CAD build for the part. Positions are in the model's coordinates, mm. Face numbers are marked on the shaded views. A direction names the side the tool comes from. Give positions to 0.01 mm unless a question says otherwise; leave off trailing zeros. Order: outer loops, then holes, each group sorted by start corner. A loop starts at its lowest first (then second) coordinate and runs counter-clockwise, first axis right, second up.
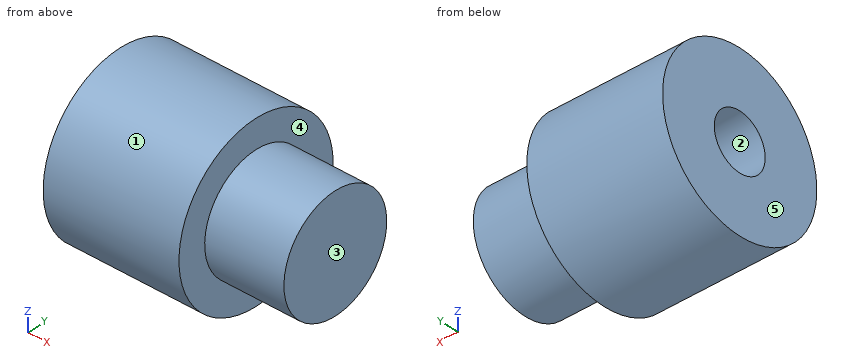
from build123d import *

# Parameters (mm, degrees)
SOCKET_1_SKETCH_W = 11.5
SOCKET_1_SKETCH_H = 4.953


with BuildPart() as part:
    # Reg_Outlet_Upper Sketch → Reg_Outlet_Upper (revolve)
    with BuildSketch(Plane.XY, mode=Mode.PRIVATE) as reg_outlet_upper_sk:
        Polygon((14, 0), (14, 10), (0, 10), (0, 15), (-24, 15), (-24, 0), align=None)
    revolve(reg_outlet_upper_sk.sketch.rotate(Axis((-1000, 0, 0), (1, 0, 0)), 90), axis=Axis((-1000, 0, 0), (1, 0, 0)))

    # Socket 1 Sketch → Socket 1 (revolve, cut)
    with BuildSketch(Plane.XY, mode=Mode.PRIVATE) as socket_1_sk:
        with Locations((-19.25, 2.4765)):
            Rectangle(SOCKET_1_SKETCH_W, SOCKET_1_SKETCH_H)
    revolve(socket_1_sk.sketch.rotate(Axis((-1000, 0, 0), (1, 0, 0)), 90), axis=Axis((-1000, 0, 0), (1, 0, 0)), mode=Mode.SUBTRACT)


solid = part.part
1. Wall check: line 1 (Y direction, x = -17.25, z = 0); line 2 (X direction, y = -4.75, z = -9.75); line 3 (Z direction, x = -22, y = 0.75). Give the ranges that are in metal, low to high.
2. Pin check, flat tips, straight feed: P1, Ø2, axis at x = 7.5, y = 6, coming from the +Z side; P2, Ø3, axis at y = 2, z = 11.5, coming from the +X side; P3, Ø5, axis at x = -9, z = 7.5, coming from the -Y side. Stop position of each tip, or through.
3. Saw through at A-A on z = 0. Give the cut face in (x, y).
4. 3-axis set-ups, long thin cutter, end or side, ignore diameter. For the marked faces 4 and 5: which of +Z, -Z, +X, -X, +Y, -Y reach the whole face in a straight line?
5. Saw through at C-C on x = 11.5. Give the cut face in (y, z).
6. Mould opens along Y. For the marked faces 1, 2 and 3 say: released by +Y, released by -Y, zero draft, split by the parting line, or undercut.
7. Saw through at D-D on x = -19.5. Give the cut face in (y, z).
Reported:
1. line 1: y = -15 to -4.95, 4.95 to 15
1. line 2: x = -24 to 0
1. line 3: z = -14.98 to -4.9, 4.9 to 14.98
2. P1: stops at z = 8.66
2. P2: stops at x = 0
2. P3: stops at y = -14.14
3. outline: (-24, -15) - (0, -15) - (0, -10) - (14, -10) - (14, 10) - (0, 10) - (0, 15) - (-24, 15) - (-24, 4.95) - (-13.5, 4.95) - (-13.5, -4.95) - (-24, -4.95) - close
4. face 4: +X
4. face 5: +Z, -Z, -X, +Y, -Y
5. outline: circle Ø20 at (0, 0)
6. face 1: split by the parting line
6. face 2: undercut
6. face 3: zero draft
7. outline: circle Ø30 at (0, 0); hole circle Ø9.91 at (0, 0)
